Here's the drawing with two shaded views (mm, measured from the low corner). I have some questions. Give positions to 0.01 mm unless a question says otherwise; leave off trailing zeros. Order: outer loops, then holes, each group sorted by start corner. A loop starts at its lowest first (then second) coordinate and runs counter-clockwise, first axis right, second up. Notation, with made-up numbers: M 23.25,-30 L 62.25,-30 A24 cw 62.25,-6 Z; hole C -9,37.5 d9. An arc over 180 degrees is marked long. Use a Markdown table: item, result. Add a question column.
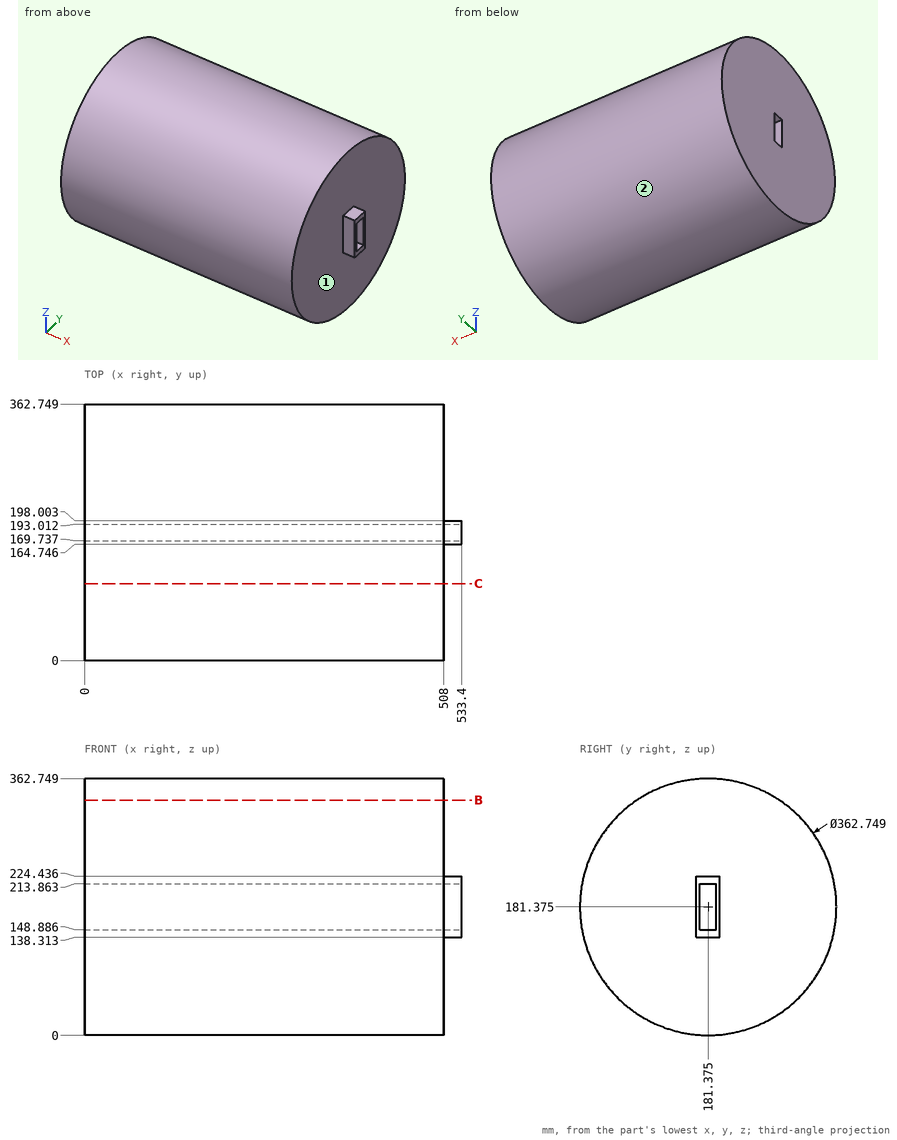
1) Suppose I cut it at B-B on z = 332.5. Please give me the cut outline in (x, y) (1 decimal), and give its area (3 significant figures).
2) Please list where these lines run through material, in increasing order: line 1 (Y direction, x = 509, z = 174); line 2 (Z direction, x = 282.5, y = 183); line 3 (Y direction, x = 117, z = 182.5) (1 decimal). Write a range as from..to.
3) Suppose I cut it at C-C on y = 109. Please give me the cut outline in (x, z) (1 decimal), and give its area (3 significant figures).
4) We'd pull the mould along Z, two halves only. Please class the marked faces 1 and 2: pulls with the +Z half, pulls with the -Z half, needs draft (parallel to the pull), parting line crosses it, or undercut.
5) For pin 1 (12 mm diameter, centred on y = 277.5, z = 231, fed in from +X); pin 2 (12.5 mm diameter, centred on x = 520.5, z = 181.5, fed in from +Y); pin 3 (1.5 mm diameter, centred on x = 436, z = 63, fed in from -Y), each with a flat end and sliding along its axis, tell me the tip position at first contact or that it passes through.
Values found:
| question | item | result |
|---|---|---|
| 1 | outline | M 0,81.1 L 508,81.1 L 508,281.7 L 0,281.7 Z |
| 1 | area | 102,000 mm^2 |
| 2 | line 1 | y = 164.75..169.74, 193.01..198 |
| 2 | line 2 | z = 0.01..148.89, 213.86..362.74 |
| 2 | line 3 | y = 0..169.7, 193..362.7 |
| 3 | outline | M 0,15.1 L 508,15.1 L 508,347.7 L 0,347.7 Z |
| 3 | area | 169,000 mm^2 |
| 4 | face 1 | needs draft |
| 4 | face 2 | parting line crosses it |
| 5 | pin 1 | stops at x = 508 |
| 5 | pin 2 | stops at y = 198 |
| 5 | pin 3 | stops at y = 43.31 |
